Geometry: final body of the model. Coordinates: model frame, mm. A direction names the side the tool comes from. Coordinates: 2 decimals unless noted, no trailing zeros. Order: outer loops, then holes, each group sorted by start corner. A loop starts at its lowest first (then second) coordinate and runs counter-clockwise, first axis right, second up. Notation, with made-up numbers: (-1.5, 49.5) - (10.5, 49.5) arc R30 ccw to (10.5, 85.5) - close; hole circle Ø3 at (-11.5, -29). An arc over 180 degrees is marked (long way). Use a Markdown table: item, result. Add a question column.
```python
from build123d import *

# Parameters (mm, degrees)
SKETCH2_R           = 21
BOSS_EXTRUDE1_DEPTH = 18


with BuildPart() as part:
    # Sketch2 → Boss-Extrude1 (new body)
    with BuildSketch(Plane.XY):
        with BuildLine():
            Line((10, 4), (43.984378813, 4))
            ThreePointArc((43.984378813, 4), (46.446208632, 4.847319563), (47.865060169, 7.03030303))
            ThreePointArc((47.865060169, 7.03030303), (105, 0), (47.865060169, -7.03030303))
            ThreePointArc((47.865060169, -7.03030303), (46.446208632, -4.847319563), (43.984378813, -4))
            Line((43.984378813, -4), (10, -4))
            ThreePointArc((10, -4), (8.242640687, -8.242640687), (4, -10))
            Line((4, -10), (4, -43.984378813))
            ThreePointArc((4, -43.984378813), (4.847319563, -46.446208632), (7.03030303, -47.865060169))
            ThreePointArc((7.03030303, -47.865060169), (0, -105), (-7.03030303, -47.865060169))
            ThreePointArc((-7.03030303, -47.865060169), (-4.847319563, -46.446208632), (-4, -43.984378813))
            Line((-4, -43.984378813), (-4, -10))
            ThreePointArc((-4, -10), (-8.242640687, -8.242640687), (-10, -4))
            Line((-10, -4), (-43.984378813, -4))
            ThreePointArc((-43.984378813, -4), (-46.446208632, -4.847319563), (-47.865060169, -7.03030303))
            ThreePointArc((-47.865060169, -7.03030303), (-105, 0), (-47.865060169, 7.03030303))
            ThreePointArc((-47.865060169, 7.03030303), (-46.446208632, 4.847319563), (-43.984378813, 4))
            Line((-43.984378813, 4), (-10, 4))
            ThreePointArc((-10, 4), (-8.242640687, 8.242640687), (-4, 10))
            Line((-4, 10), (-4, 43.984378813))
            ThreePointArc((-4, 43.984378813), (-4.847319563, 46.446208632), (-7.03030303, 47.865060169))
            ThreePointArc((-7.03030303, 47.865060169), (0, 105), (7.03030303, 47.865060169))
            ThreePointArc((7.03030303, 47.865060169), (4.847319563, 46.446208632), (4, 43.984378813))
            Line((4, 43.984378813), (4, 10))
            ThreePointArc((4, 10), (8.242640687, 8.242640687), (10, 4))
        make_face()
        with Locations((76, 0)):
            Circle(SKETCH2_R, mode=Mode.SUBTRACT)
        with Locations((0, -76)):
            Circle(SKETCH2_R, mode=Mode.SUBTRACT)
        with Locations((-76, 0)):
            Circle(SKETCH2_R, mode=Mode.SUBTRACT)
        with Locations((0, 76)):
            Circle(SKETCH2_R, mode=Mode.SUBTRACT)
    extrude(amount=BOSS_EXTRUDE1_DEPTH)


solid = part.part
```
1) Section C-C (z = 14.5). Return loops of the section in (x, y), then the cut area to 3 significant figures.
2) Draft query along X for faces 1 (the face through (0, -7, 18)), 2 (the face through (11.3, -58.3, 8.9)), 3 (the face through (1.176, -104.976, 8.874)). Return one class per face: pulls with the +X half, pulls with the -X half, needs draft (parallel to the pull), parting line crosses it, or undercut.
3) Ray query, line 1 along Y through (x, z) = (-15.5, 4.25); line 2 along Y through (x, z) = (25, 7.5); line 3 along X through (y, z) = (24, 12). Return the intervals inside material, ascending.
4) Section D-D (y = -25). Return loops of the section in (x, z), then the cut area to 3 significant figures.
5) Section A-A (x = -76). Return loops of the section in (y, z).
6) Pin query (flat end, axial travel): pin 1 (9 mm diameter, centred on x = 19.5, z = 6.5, fed in from -Y); pin 2 (3 mm diameter, centred on y = -27.5, z = 3.5, fed in from +X); pin 3 (2 mm diameter, centred on y = -84, z = 3, fed in from -X). Return the tip coordinate at first contact, or that it passes through.
7) Set-up query: faces 4 (the face through (8.196, 8.289, 8.874)), 5 (the face through (0, -7, 0)). Return all of +Z, -Z, +X, -X, +Y, -Y with unobstructed straight access to the full face (end or side cutting, diameter ignored); none if empty.
Values follow:
| question | item | result |
|---|---|---|
| 1 | outline | (-47.87, -7.03) arc R4 cw to (-43.98, -4) - (-10, -4) arc R6 ccw to (-4, -10) - (-4, -43.98) arc R4 cw to (-7.03, -47.87) arc R29 ccw (long way) to (7.03, -47.87) arc R4 cw to (4, -43.98) - (4, -10) arc R6 ccw to (10, -4) - (43.98, -4) arc R4 cw to (47.87, -7.03) arc R29 ccw (long way) to (47.87, 7.03) arc R4 cw to (43.98, 4) - (10, 4) arc R6 ccw to (4, 10) - (4, 43.98) arc R4 cw to (7.03, 47.87) arc R29 ccw (long way) to (-7.03, 47.87) arc R4 cw to (-4, 43.98) - (-4, 10) arc R6 ccw to (-10, 4) - (-43.98, 4) arc R4 cw to (-47.87, 7.03) arc R29 ccw (long way) to start; hole circle Ø42 at (-76, 0); hole circle Ø42 at (0, -76); hole circle Ø42 at (0, 76); hole circle Ø42 at (76, 0) |
| 1 | area | 6,600 mm² |
| 2 | face 1 | needs draft |
| 2 | face 2 | undercut |
| 2 | face 3 | parting line crosses it |
| 3 | line 1 | y = -100.51 to -90.17, -61.83 to -51.49, -4 to 4, 51.49 to 61.83, 90.17 to 100.51 |
| 3 | line 2 | y = -90.7 to -61.3, -4 to 4, 61.3 to 90.7 |
| 3 | line 3 | x = -92.28 to -59.72, -4 to 4, 59.72 to 92.28 |
| 4 | outline | (-90.7, 0) - (-61.3, 0) - (-61.3, 18) - (-90.7, 18) - close; (-4, 0) - (4, 0) - (4, 18) - (-4, 18) - close; (61.3, 0) - (90.7, 0) - (90.7, 18) - (61.3, 18) - close |
| 4 | area | 1,200 mm² |
| 5 | outline | (-29, 0) - (-21, 0) - (-21, 18) - (-29, 18) - close; (21, 0) - (29, 0) - (29, 18) - (21, 18) - close |
| 6 | pin 1 | stops at y = -100.82 |
| 6 | pin 2 | stops at x = 88.85 |
| 6 | pin 3 | stops at x = -28.14 |
| 7 | face 4 | +Z, -Z |
| 7 | face 5 | -Z, +X, -X, +Y, -Y |
